from build123d import *

# Parameters (mm, degrees)
SKETCH1_W           = 330.2
SKETCH1_H           = 469.9
SKETCH1_R           = 8.6487
BOSS_EXTRUDE1_DEPTH = 25.4


with BuildPart() as part:
    # Sketch1 → Boss-Extrude1 (new body)
    with BuildSketch(Plane(origin=(0, 0, 0), x_dir=(1, 0, 0), z_dir=(0, 1, 0))):
        with Locations((-165.1, 234.95)):
            Rectangle(SKETCH1_W, SKETCH1_H)
        with Locations((-165.1, 444.5)):
            Circle(SKETCH1_R, mode=Mode.SUBTRACT)
        with Locations((-25.4, 234.95)):
            Circle(SKETCH1_R, mode=Mode.SUBTRACT)
        with Locations((-165.1, 25.4)):
            Circle(SKETCH1_R, mode=Mode.SUBTRACT)
        with Locations((-304.8, 234.95)):
            Circle(SKETCH1_R, mode=Mode.SUBTRACT)
        with Locations((-88.9, 101.6)):
            Circle(SKETCH1_R, mode=Mode.SUBTRACT)
        with Locations((-88.9, 152.4)):
            Circle(SKETCH1_R, mode=Mode.SUBTRACT)
        with Locations((-88.9, 203.2)):
            Circle(SKETCH1_R, mode=Mode.SUBTRACT)
        with Locations((-88.9, 254)):
            Circle(SKETCH1_R, mode=Mode.SUBTRACT)
        with Locations((-241.3, 101.6)):
            Circle(SKETCH1_R, mode=Mode.SUBTRACT)
        with Locations((-241.3, 152.4)):
            Circle(SKETCH1_R, mode=Mode.SUBTRACT)
        with Locations((-241.3, 203.2)):
            Circle(SKETCH1_R, mode=Mode.SUBTRACT)
        with Locations((-241.3, 254)):
            Circle(SKETCH1_R, mode=Mode.SUBTRACT)
    extrude(amount=BOSS_EXTRUDE1_DEPTH)


solid = part.part
Here's how the part is built. I have some questions about the finished solid (model axes, mm). Round coordinates to 2 decimals unless told otherwise and drop trailing zeros. Order: outer loops, then holes, each group sorted by start corner. A loop starts at its lowest first (then second) coordinate and runs counter-clockwise, first axis right, second up. Notation, with made-up numbers: M 44,-23.5 L 92,-23.5 A27 cw 92,-0.5 Z; hole C 32,-24 d11. An arc over 180 degrees is marked long. Return JSON: item names as keys, results as strings. Group by question number.
1. Please list where these lines run through material, in increasing order: probe 1 along X at (y, z) = (20.25, -203.2); probe 2 along Z at (x, y) = (-165.1, 7.25); probe 3 along Z at (x, y) = (-88.9, 19.25).
2. If we mould it in two halves opening along Z, with no side actions, what happens to faces 1 (the face through (-249.94, 12.52, -101.98)), 2 (the face through (-97.54, 12.52, -152.78)), 3 (the face through (-167, 13, 0)), 4 (the face through (-330.2, 13, -232))? For each: pulls with the +Z half, pulls with the -Z half, needs draft (parallel to the pull), parting line crosses it, or undercut.
3. I'm going to push flat-ended pins straight in: pin 1 Ø20 at (x, z) = (-241.3, -203.2) entering from -Y; pin 2 Ø15.5 at (x, z) = (-241.3, -254) entering from -Y. Where does each tip first touch, or does it pass through?
4. If we section it at B-B on x = -241.3: List the corners of the cut face in (y, z) for me, then the cut area to 3 significant figures.
5. If we section it at A-A on z = -444.5: List the corners of the cut face in (x, y) for me.
6. If we section it at C-C on z = -254: List the corners of the cut face in (x, y) for me.
7. If we section it at D-D on x = -304.8: List the corners of the cut face in (y, z) for me.
Reply:
{
 "1": {"probe 1": "-330.2 to -249.95, -232.65 to -97.55, -80.25 to 0", "probe 2": "-469.9 to -453.15, -435.85 to -34.05, -16.75 to 0", "probe 3": "-469.9 to -262.65, -245.35 to -211.85, -194.55 to -161.05, -143.75 to -110.25, -92.95 to 0"},
 "2": {"face 1": "undercut", "face 2": "undercut", "face 3": "pulls with the +Z half", "face 4": "needs draft"},
 "3": {"pin 1": "y = 0", "pin 2": "through"},
 "4": {"outline": "M 0,-469.9 L 25.4,-469.9 L 25.4,-262.65 L 0,-262.65 Z; M 0,-245.35 L 25.4,-245.35 L 25.4,-211.85 L 0,-211.85 Z; M 0,-194.55 L 25.4,-194.55 L 25.4,-161.05 L 0,-161.05 Z; M 0,-143.75 L 25.4,-143.75 L 25.4,-110.25 L 0,-110.25 Z; M 0,-92.95 L 25.4,-92.95 L 25.4,0 L 0,0 Z", "area": "10,200 mm^2"},
 "5": {"outline": "M -330.2,0 L -173.75,0 L -173.75,25.4 L -330.2,25.4 Z; M -156.45,0 L 0,0 L 0,25.4 L -156.45,25.4 Z"},
 "6": {"outline": "M -330.2,0 L -249.95,0 L -249.95,25.4 L -330.2,25.4 Z; M -232.65,0 L -97.55,0 L -97.55,25.4 L -232.65,25.4 Z; M -80.25,0 L 0,0 L 0,25.4 L -80.25,25.4 Z"},
 "7": {"outline": "M 0,-469.9 L 25.4,-469.9 L 25.4,-243.6 L 0,-243.6 Z; M 0,-226.3 L 25.4,-226.3 L 25.4,0 L 0,0 Z"}
}
